```python
from build123d import *

# Parameters (mm, degrees)
SKETCH1_W               = 16
SKETCH1_H               = 18
SKETCH1_W_2             = 12
SKETCH1_H_2             = 14
EXTRUDE_THIN1_DEPTH     = 4
BOSS_EXTRUDE1_DEPTH     = 2
SKETCH3_R               = 3
BOSS_EXTRUDE2_DEPTH     = 2
BOSS_EXTRUDE2_TAPER     = 35
BOSS_EXTRUDE3_DEPTH     = 2.2
CUT_EXTRUDE4_REACH      = 35.62
SKETCH10_W              = 0.2
SKETCH10_H              = 25.531461486
SKETCH5_R               = 3
CUT_EXTRUDE1_DEPTH      = 2
CUT_EXTRUDE1_DRAFT      = -35
MIRROR3_COPY_1_SKETCH_R = 3
MIRROR3_COPY_1_DEPTH    = 2
MIRROR3_COPY_1_DRAFT    = -35
SKETCH13_W              = 12
SKETCH13_H              = 1
BOSS_EXTRUDE4_DEPTH     = 8
CUT_EXTRUDE5_REACH      = 35.396
SKETCH11_R              = 0.5


with BuildPart() as part:
    # Sketch1 → Extrude-Thin1 (new, symmetric)
    with BuildSketch(Plane.XY):
        Rectangle(SKETCH1_W, SKETCH1_H)
        Rectangle(SKETCH1_W_2, SKETCH1_H_2, mode=Mode.SUBTRACT)
    extrude_thin1 = extrude(amount=EXTRUDE_THIN1_DEPTH, both=True)

    # Sketch2 → Boss-Extrude1 (add)
    with BuildSketch(Plane(origin=(8, 0, 0), x_dir=(0, 0, -1), z_dir=(1, 0, 0))):
        with BuildLine():
            Line((0, 9), (-17.5, 9))
            ThreePointArc((-17.5, 9), (-26.5, 0), (-17.5, -9))
            Line((-17.5, -9), (0, -9))
            Line((0, -9), (0, 9))
        make_face()
    boss_extrude1 = extrude(amount=-BOSS_EXTRUDE1_DEPTH)

    # Sketch3 → Boss-Extrude2 (add)
    with BuildSketch(Plane(origin=(8, 0, 0), x_dir=(0, 0, -1), z_dir=(1, 0, 0))):
        with Locations((-17.5, 0)):
            Circle(SKETCH3_R)
    boss_extrude2 = extrude(amount=BOSS_EXTRUDE2_DEPTH, taper=BOSS_EXTRUDE2_TAPER)

    # Sketch4 → Boss-Extrude3 (add)
    with BuildSketch(Plane(origin=(8, 0, 0), x_dir=(0, 0, -1), z_dir=(1, 0, 0))):
        with BuildLine():
            Line((0, 9), (17.5, 9))
            ThreePointArc((17.5, 9), (26.5, 0), (17.5, -9))
            Line((17.5, -9), (0, -9))
            Line((0, -9), (0, 9))
        make_face()
    boss_extrude3 = extrude(amount=BOSS_EXTRUDE3_DEPTH)

    # Sketch10 → Cut-Extrude4 (cut, up to next)
    with BuildSketch(Plane(origin=(0, 9, 0), x_dir=(1, 0, 0), z_dir=(0, 1, 0)), mode=Mode.PRIVATE) as cut_extrude4_sk1:
        with Locations((8.1, 16.765730743)):
            Rectangle(SKETCH10_W, SKETCH10_H)
    cut_extrude4_tool1 = extrude(cut_extrude4_sk1.sketch, amount=-CUT_EXTRUDE4_REACH, mode=Mode.PRIVATE) & part.part
    cut_extrude4 = cut_extrude4_tool1.solids().sort_by_distance((8.1, 9, -16.765731))[0]
    add(cut_extrude4, mode=Mode.SUBTRACT)


with BuildPart() as cut_extrude1_tool:
    # Sketch5 → Cut-Extrude1 (with draft: the straight prism first)
    with BuildSketch(Plane.ZY.offset(-8.2)):
        with Locations((-17.5, 0)):
            Circle(SKETCH5_R)
    extrude(amount=-CUT_EXTRUDE1_DEPTH)
    # Cut-Extrude1: the draft: its side faces are tilted about the plane it starts from
    cut_extrude1_sides = [cut_extrude1_tool.faces().sort_by_distance(p)[0] for p in [
        (9.2, 0, -20.5),
    ]]
    draft(cut_extrude1_sides, Plane.ZY.offset(-8.2), CUT_EXTRUDE1_DRAFT)


with BuildPart() as part_1:
    add(part.part)

    # Cut-Extrude1: cut by cut_extrude1_tool
    add(cut_extrude1_tool.part, mode=Mode.SUBTRACT)

    # Mirror3: Extrude-Thin1, Boss-Extrude1, Boss-Extrude2, Boss-Extrude3, Cut-Extrude4 across plane
    add(extrude_thin1.mirror(Plane(origin=(0, 0, 0), x_dir=(0, 0, 1), z_dir=(1, 0, 0))))
    add(boss_extrude1.mirror(Plane(origin=(0, 0, 0), x_dir=(0, 0, 1), z_dir=(1, 0, 0))))
    add(boss_extrude2.mirror(Plane(origin=(0, 0, 0), x_dir=(0, 0, 1), z_dir=(1, 0, 0))))
    add(boss_extrude3.mirror(Plane(origin=(0, 0, 0), x_dir=(0, 0, 1), z_dir=(1, 0, 0))))
    add(cut_extrude4.mirror(Plane(origin=(0, 0, 0), x_dir=(0, 0, 1), z_dir=(1, 0, 0))), mode=Mode.SUBTRACT)


with BuildPart() as mirror3_copy_1_tool:
    # Mirror3 copy 1 sketch → Mirror3 copy 1 (with draft: the straight prism first)
    with BuildSketch(Plane(origin=(-8.2, 0, 0), x_dir=(0, 0, 1), z_dir=(1, 0, 0))):
        with Locations((-17.5, 0)):
            Circle(MIRROR3_COPY_1_SKETCH_R)
    extrude(amount=-MIRROR3_COPY_1_DEPTH)
    # Mirror3 copy 1: the draft: its side faces are tilted about the plane it starts from
    mirror3_copy_1_sides = [mirror3_copy_1_tool.faces().sort_by_distance(p)[0] for p in [
        (-9.2, 0, -20.5),
    ]]
    draft(mirror3_copy_1_sides, Plane(origin=(-8.2, 0, 0), x_dir=(0, 0, 1), z_dir=(1, 0, 0)), MIRROR3_COPY_1_DRAFT)


with BuildPart() as part_2:
    add(part_1.part)

    # Mirror3 copy 1: cut by mirror3_copy_1_tool
    add(mirror3_copy_1_tool.part, mode=Mode.SUBTRACT)

    # Sketch13 → Boss-Extrude4 (add)
    with BuildSketch(Plane.XY.offset(4)):
        with Locations((0, 6.5)):
            Rectangle(SKETCH13_W, SKETCH13_H)
    boss_extrude4 = extrude(amount=-BOSS_EXTRUDE4_DEPTH)

    # Mirror5: Boss-Extrude4 across plane
    add(boss_extrude4.mirror(Plane.ZX))

    # Sketch11 → Cut-Extrude5 (cut, up to next)
    with BuildSketch(Plane.XY.offset(4), mode=Mode.PRIVATE) as cut_extrude5_sk1:
        with Locations((0, 7.5)):
            Circle(SKETCH11_R)
    cut_extrude5_tool1 = extrude(cut_extrude5_sk1.sketch, amount=-CUT_EXTRUDE5_REACH, mode=Mode.PRIVATE) & part_2.part
    cut_extrude5 = cut_extrude5_tool1.solids().sort_by_distance((0, 7.5, 4))[0]
    add(cut_extrude5, mode=Mode.SUBTRACT)

    # Mirror4: Cut-Extrude5 across plane
    add(cut_extrude5.mirror(Plane.ZX), mode=Mode.SUBTRACT)


solid = part_2.part
```
For this review, take the finished solid that the model builds, in its own axes (mm). A direction names the side the tool comes from. Round coordinates to 2 decimals unless told otherwise and drop trailing zeros. Write each loop counter-clockwise with the first axis right and the second up, starting at its lowest first coordinate (ties: lowest second). Pieces come first, ordered by that corner, then holes. Notation, with made-up numbers: M 48,33.25 L 99,33.25 A22 cw 99,51.25 Z; hole C 62.25,-11 d6. An arc over 180 degrees is marked long. One line per item, written item: value. Start each with the question number.
(1) Machinability: for faces 1 (the flat face through (8.2, 0, -13)), 2 (the flat face through (-0.08, -6.85, 4)), 3 (the flat face through (10, 0, 18)), 4 (the flat face through (-10, 0, 18)), which of the approach directions +Z, -Z, +X, -X, +Y, -Y give a long, thin tool a straight path to every point of the face, cutting with its end or side? Answer none if there is none.
(2) Wall thickness on line 1 (Y direction, x = 0, z = -0.25); line 2 (X direction, y = 2.5, z = -2); line 3 (X direction, y = -2, z = 4.5): over which ranges is each line inside the solid? List them lowest first.
(3) Insertion check: pin 1 (1.1 mm diameter, centred on x = 9.5, y = -2, fed in from +Z); pin 2 (4 mm diameter, centred on y = -2.5, z = 12.5, fed in from +X); pin 3 (1 mm diameter, centred on y = 1, z = 17.5, fed in from +X). Each pin has a flat end and moves straight along its axis. Give the tip position at first contact, or say it passes through.
(4) We need section C-C (y = -4.5). Give the boundary of the cut face in (x, z), and give its area (3 significant figures).
(5) We need section B-B (z = -3). Give the boundary of the cut face in (x, y).
(6) The part is to be moulded in two halves that separate along Y. For faces 5 (the flat face through (-8.2, 0, -13)), 6 (the cylindrical face through (-7.014, 0.198, 26.498)), 7 (the flat face through (6, 0, 11)), say which applies: released by +Y, released by -Y, zero draft, split by the parting line, or undercut.
(7) We need section A-A (z = 8). Give the boundary of the cut face in (x, y).
(8) We need section D-D (x = -4). Give the boundary of the cut face in (y, z).
Result:
1. face 1: -Z, +Y, -Y
1. face 2: +Z, +Y, -Y
1. face 3: +Z, +X, +Y, -Y
1. face 4: +Z, -X, +Y, -Y
2. line 1: -9 to -8, -7 to -6, 6 to 7, 8 to 9
2. line 2: -10.2 to -6, 6 to 10.2
2. line 3: -8 to -6, 6 to 8
3. pin 1: z = 19.03
3. pin 2: x = 8
3. pin 3: x = 10
4. outline: M -10.2,-25.29 L -8.2,-25.29 L -8.2,-4 L -6,-4 L -6,25.29 L -8,25.29 L -8,0 L -10.2,0 Z; M 6,-4 L 8.2,-4 L 8.2,-25.29 L 10.2,-25.29 L 10.2,0 L 8,0 L 8,25.29 L 6,25.29 Z
4. area: 220 mm²
5. outline: M -10.2,-9 L 10.2,-9 L 10.2,9 L -10.2,9 Z; hole M -6,-6 L 6,-6 L 6,6 L -6,6 Z; hole C 0,-7.5 d1; hole C 0,7.5 d1
6. face 5: zero draft
6. face 6: split by the parting line
6. face 7: undercut
7. outline: M -8,-9 L -6,-9 L -6,9 L -8,9 Z; M 6,-9 L 8,-9 L 8,9 L 6,9 Z
8. outline: M -9,-4 L -6,-4 L -6,4 L -9,4 Z; M 6,-4 L 9,-4 L 9,4 L 6,4 Z
